```python
from build123d import *

# Parameters (mm, degrees)
BOSS_EXTRU_1_DEPTH         = 300
ESQUISSE2_R                = 2.5
ENL_V_MAT_EXTRU_1_DEPTH    = 301.430108345
R_P_TITION_LIN_AIRE1_COUNT = 9
R_P_TITION_LIN_AIRE1_PITCH = 67


with BuildPart() as part:
    # Esquisse1 → Boss.-Extru.1 (new, symmetric)
    with BuildSketch(Plane.XY):
        with BuildLine():
            Line((16, -1.5), (0, -1.5))
            ThreePointArc((0, -1.5), (-1.060660172, 1.060660172), (1.5, 0))
            Line((1.5, 0), (16, 0))
            Line((16, 0), (16, -1.5))
        make_face()
    extrude(amount=BOSS_EXTRU_1_DEPTH, both=True)

    # Esquisse2 → Enlèv. mat.-Extru.1 (cut, through all)
    with BuildSketch(Plane(origin=(0, 0, 0), x_dir=(1, 0, 0), z_dir=(0, 1, 0))):
        with Locations(Location((8.75, -268, 0), (0, 0, 180))):
            Circle(ESQUISSE2_R)
    enl_v_mat_extru_1 = extrude(amount=-ENL_V_MAT_EXTRU_1_DEPTH, mode=Mode.SUBTRACT)

    # Répétition linéaire1: Enlèv. mat.-Extru.1 ×9
    with Locations(*[(0, 0, -i * R_P_TITION_LIN_AIRE1_PITCH) for i in range(1, R_P_TITION_LIN_AIRE1_COUNT)]):
        add(enl_v_mat_extru_1, mode=Mode.SUBTRACT)


solid = part.part
```
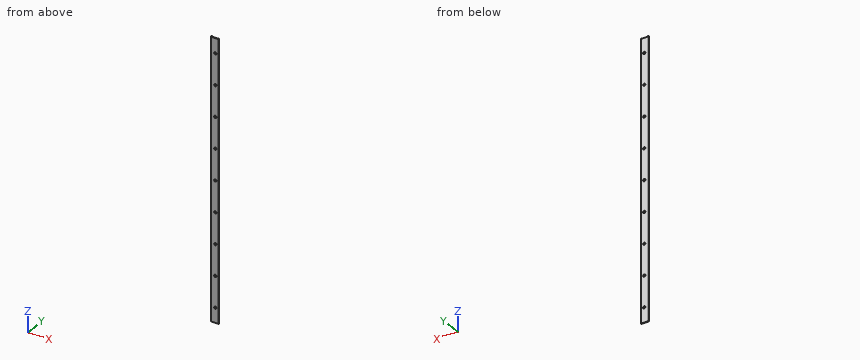
Geometry: final body of the model. Coordinates: model frame, mm. Coordinates: 2 decimals unless noted, no trailing zeros. Order: outer loops, then holes, each group sorted by start corner. A loop starts at its lowest first (then second) coordinate and runs counter-clockwise, first axis right, second up. Notation, with made-up numbers: (17, 87) - (74, 87) arc R29 cw to (74, 119) - close; hole circle Ø6 at (41.25, 74). An arc over 180 degrees is marked (long way). Return JSON: item names as keys, results as strings. Group by question number.
1. Cut plane A-A (y = -0.55). Count the separate pieces of the cut face and the enclosed holes in it, plus the area to 3 significant figures.
2. Pin query (flat end, axial travel): pin 1 (5 mm diameter, centred on x = 3.5, z = 67.5, fed in from +Y); pin 2 (6.5 mm diameter, centred on x = 8.75, z = -67, fed in from +Y); pin 3 (1.5 mm diameter, centred on y = -1, z = -172, fed in from -X). Return the tip coordinate at first contact, or that it passes through.
3. Material intervals for line 1 along Y through (x, z) = (3, -250.5); line 2 along X through (y, z) = (-0.45, -217); line 3 along X through (y, z) = (-0.3, 242.5), sorted ascending. Write a range as [from, to].
4. Cut plane B-B (z = -83). Output: boundary loops of the cut face in (x, y), plus the area to 3 significant figures.
Resolved:
{
 "1": {"separate pieces": "1", "enclosed holes": "9", "area": "10,300 mm²"},
 "2": {"pin 1": "stops at y = 1.12", "pin 2": "stops at y = 0", "pin 3": "stops at x = -1.48"},
 "3": {"line 1": "y = [-1.5, 0]", "line 2": "x = [-1.43, 16]", "line 3": "x = [-1.47, 16]"},
 "4": {"outline": "(0, -1.5) - (16, -1.5) - (16, 0) - (1.5, 0) arc R1.5 ccw (long way) to start", "area": "29.3 mm²"}
}
